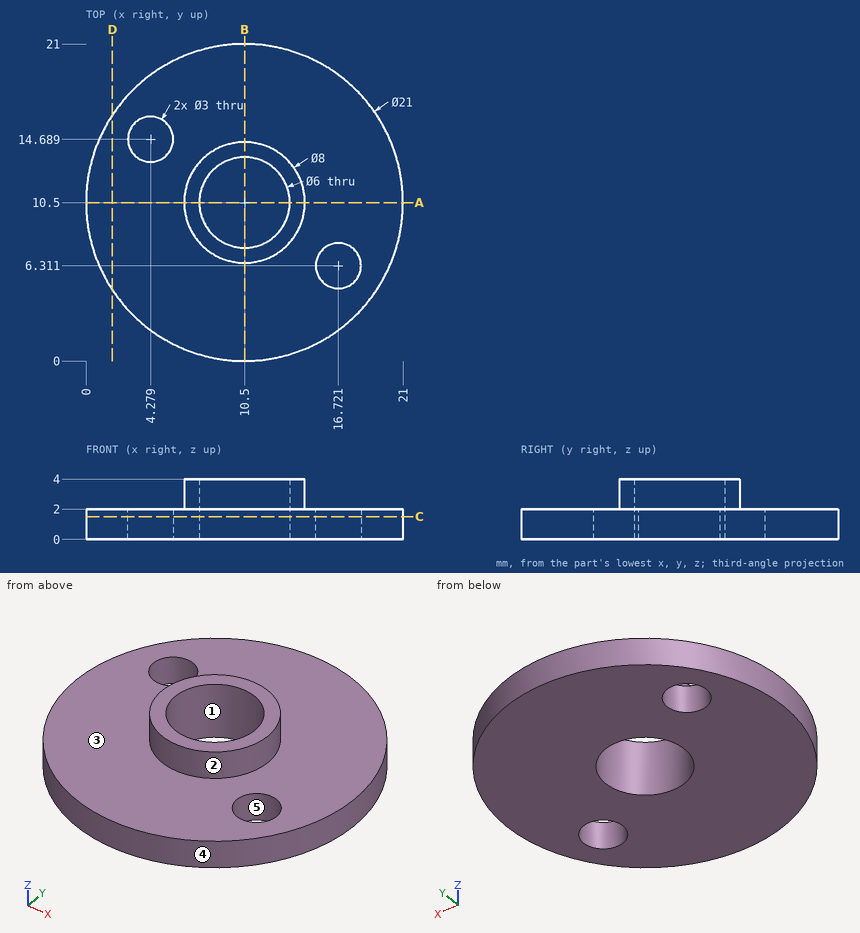
Input: dimensioned drawing with shaded views. Units: mm. Origin: part minimum x, y, z. A direction names the side the tool comes from. Give positions to 0.01 mm unless a question says otherwise; leave off trailing zeros. Loops run counter-clockwise (first coordinate to the right, second up) from the corner with the lowest first, then second, coordinate; pieces in that order, holes last. Notation, with made-up numbers: M 60.5,28 L 85.5,28 A22 cw 85.5,42 Z; hole C 58.25,-39.75 d8. An arc over 180 degrees is marked long. Put each result on its own line as item: value.
1) Cut plane A-A, the plane y = 10.5. Return the cut outline in (x, z).
Computed values:
outline: M 0,0 L 7.5,0 L 7.5,4 L 6.5,4 L 6.5,2 L 0,2 Z; M 13.5,0 L 21,0 L 21,2 L 14.5,2 L 14.5,4 L 13.5,4 Z
2) Cut plane C-C, the plane z = 1.5. Return the cut outline in (x, y).
Computed values:
outline: C 10.5,10.5 d21; hole C 4.28,14.69 d3; hole C 10.5,10.5 d6; hole C 16.72,6.31 d3
3) First-contact query: P1, Ø1.5, axis at x = 15.5, y = 11, coming from the +Z side; P2, Ø1.5, axis at y = 18, z = 1.5, coming from the +X side; P3, Ø1, axis at y = 9.5, z = 1, coming from the +X side. Flat tips, straight axial feed; report the tip coordinate or a pass-through.
Computed values:
P1: stops at z = 2
P2: stops at x = 18.54
P3: stops at x = 20.99
4) Reachability of the marked faces 1 and 2 from +Z, -Z, +X, -X, +Y, -Y: full face, straight path, thin tool, end or side. Return the list, or none.
Computed values:
face 1: +Z, -Z
face 2: +Z
5) Cut plane D-D, the plane x = 1.75. Return the cut outline in (y, z).
Computed values:
outline: M 4.7,0 L 16.3,0 L 16.3,2 L 4.7,2 Z
6) Mould query, pull axis X, two halves, no side actions, for the marked faces 3, 4 and 5. Classes: released by +X, released by -X, zero draft, split by the parting line, or undercut.
Computed values:
face 3: zero draft
face 4: split by the parting line
face 5: undercut
7) Material intervals for L1, parallel to Y at x = 10.5, z = 1.3; L2, parallel to Z at x = 8.75, y = 6.25; L3, parallel to X at y = 13.25, z = 3.4 (1 decimal), sorted ascending. Write a range as from..to.
Computed values:
L1: y = 0..7.5, 13.5..21
L2: z = 0..2
L3: x = 7.6..9.3, 11.7..13.4
